Can you work these out from the drawing? Everything is in mm from the part's minimum corner. A direction names the side the tool comes from. Give positions to 0.01 mm unless a question says otherwise; leave off trailing zeros. Loops run counter-clockwise (first coordinate to the right, second up) from the corner with the lowest first, then second, coordinate; pieces in that order, holes last. Notation, with made-up numbers: (20, 5) - (61, 5) arc R13 ccw to (61, 14) - close; hole circle Ø2 at (81, 88.5). An arc over 180 degrees is marked (long way). Answer in a Markdown table with one row per item.
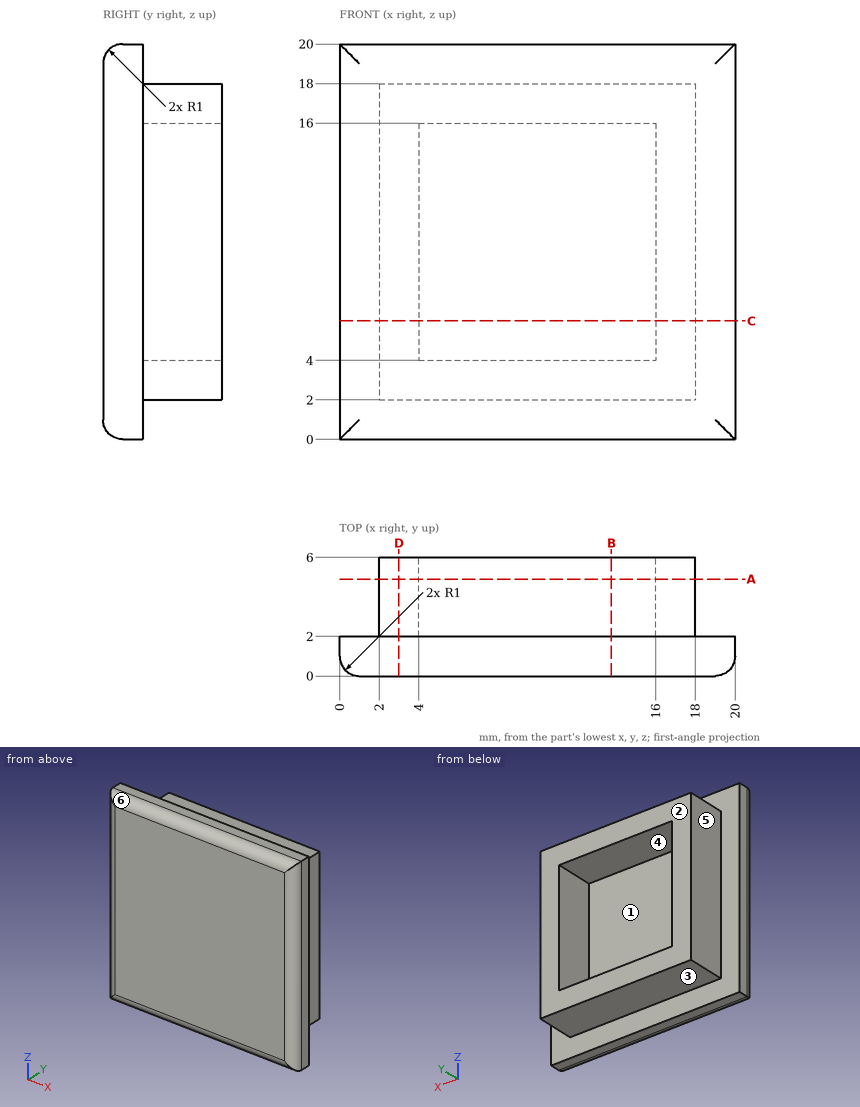
Q1. For pin 1 (2 mm diameter, centred on x = 9.5, y = 2.5, fed in from -Z); pin 2 (9.5 mm diameter, centred on x = 11, z = 9.5, fed in from +Y); pin 3 (1.5 mm diameter, centred on x = 10, y = 3, fed in from +Z); pin 4 (1.2 mm diameter, centred on x = 6.5, y = 5, fed in from -Z), each with a flat end and sliding along its axis, tell me the tip position at first contact or that it passes through.
Checked values:
| item | result |
|---|---|
| pin 1 | stops at z = 0 |
| pin 2 | stops at y = 2 |
| pin 3 | stops at z = 18 |
| pin 4 | stops at z = 2 |
Q2. If I drill on line 1 (X direction, y = 3.95, z = 10.5); line 2 (Y direction, x = 1, z = 17.5), over which ranges is the centre line in solid material (lowest first)? Write a range as [from, to].
Checked values:
| item | result |
|---|---|
| line 1 | x = [2, 4], [16, 18] |
| line 2 | y = [0, 2] |
Q3. On a 3-axis mill with a long thin cutter (end or side, diameter ignored), from which of +Z, -Z, +X, -X, +Y, -Y can I reach the whole of each face in a straight line? I mean the marked faces 1, 2 and 3. Say none if no direction works.
Checked values:
| item | result |
|---|---|
| face 1 | +Y |
| face 2 | +Z, -Z, +X, -X, +Y |
| face 3 | -Z, +X, -X, +Y |
Q4. Imagine slicing it at A-A, the plane y = 4.9. Write out the boundary of the cut face in (x, z), and give its area (3 significant figures).
Checked values:
| item | result |
|---|---|
| outline | (2, 2) - (18, 2) - (18, 18) - (2, 18) - close; hole (4, 4) - (16, 4) - (16, 16) - (4, 16) - close |
| area | 112 mm² |
Q5. Imagine slicing it at D-D, the plane x = 3. Write out the boundary of the cut face in (y, z).
Checked values:
| item | result |
|---|---|
| outline | (0, 1) arc R1 ccw to (1, 0) - (2, 0) - (2, 2) - (6, 2) - (6, 18) - (2, 18) - (2, 20) - (1, 20) arc R1 ccw to (0, 19) - close |
Q6. If we mould it in two halves opening along X, with no side actions, what happens to the marked faces 4, 5 and 6? For each: released by +X, released by -X, zero draft, split by the parting line, or undercut.
Checked values:
| item | result |
|---|---|
| face 4 | undercut |
| face 5 | released by -X |
| face 6 | zero draft |
Q7. Imagine slicing it at B-B, the plane x = 13.75. Write out the boundary of the cut face in (y, z), and give its area (3 significant figures).
Checked values:
| item | result |
|---|---|
| outline | (0, 1) arc R1 ccw to (1, 0) - (2, 0) - (2, 2) - (6, 2) - (6, 4) - (2, 4) - (2, 16) - (6, 16) - (6, 18) - (2, 18) - (2, 20) - (1, 20) arc R1 ccw to (0, 19) - close |
| area | 55.6 mm² |
Q8. Imagine slicing it at C-C, the plane z = 6. Write out the boundary of the cut face in (x, y), and give its area (3 significant figures).
Checked values:
| item | result |
|---|---|
| outline | (0, 1) arc R1 ccw to (1, 0) - (19, 0) arc R1 ccw to (20, 1) - (20, 2) - (18, 2) - (18, 6) - (16, 6) - (16, 2) - (4, 2) - (4, 6) - (2, 6) - (2, 2) - (0, 2) - close |
| area | 55.6 mm² |
